from build123d import *

# Parameters (mm, degrees)
F1_DEPTH = 25


with BuildPart() as f1:
    # F0 (on Front) → F1 (new body)
    with BuildSketch(Plane.XZ):
        with BuildLine():
            Line((5, 30.5941170816), (5, 39.686269666))
            ThreePointArc((5, 39.686269666), (2.5049165017, 39.9214903695), (0, 40))
            Line((0, 40), (0, 31))
            ThreePointArc((0, 31), (2.5082235219, 30.8983626551), (5, 30.5941170816))
        make_face()
        with BuildLine():
            Line((0, 31), (0, 40))
            ThreePointArc((0, 40), (-2.5049165017, 39.9214903695), (-5, 39.686269666))
            Line((-5, 39.686269666), (-5, 30.5941170816))
            ThreePointArc((-5, 30.5941170816), (-2.5082235219, 30.8983626551), (0, 31))
        make_face()
        with BuildLine():
            Line((-5, 30.5941170816), (-5, 39.686269666))
            ThreePointArc((-5, 39.686269666), (-28.2842712475, 28.2842712475), (-39.686269666, 5))
            Line((-39.686269666, 5), (-30.5941170816, 5))
            ThreePointArc((-30.5941170816, 5), (-21.9203102168, 21.9203102168), (-5, 30.5941170816))
        make_face()
        with BuildLine():
            Line((-30.5941170816, 5), (-39.686269666, 5))
            ThreePointArc((-39.686269666, 5), (-39.9214903695, 2.5049165017), (-40, 0))
            Line((-40, 0), (-31, 0))
            ThreePointArc((-31, 0), (-30.8983626551, 2.5082235219), (-30.5941170816, 5))
        make_face()
        with BuildLine():
            ThreePointArc((-40, 0), (-39.9214903695, -2.5049165017), (-39.686269666, -5))
            Line((-39.686269666, -5), (-30.5941170816, -5))
            ThreePointArc((-30.5941170816, -5), (-30.8983626551, -2.5082235219), (-31, 0))
            Line((-31, 0), (-40, 0))
        make_face()
        with BuildLine():
            ThreePointArc((-39.686269666, -5), (-28.2842712475, -28.2842712475), (-5, -39.686269666))
            Line((-5, -39.686269666), (-5, -30.5941170816))
            ThreePointArc((-5, -30.5941170816), (-21.9203102168, -21.9203102168), (-30.5941170816, -5))
            Line((-30.5941170816, -5), (-39.686269666, -5))
        make_face()
        with BuildLine():
            ThreePointArc((-5, -39.686269666), (-2.5049165017, -39.9214903695), (0, -40))
            Line((0, -40), (0, -31))
            ThreePointArc((0, -31), (-2.5082235219, -30.8983626551), (-5, -30.5941170816))
            Line((-5, -30.5941170816), (-5, -39.686269666))
        make_face()
        with BuildLine():
            ThreePointArc((0, -40), (2.5049165017, -39.9214903695), (5, -39.686269666))
            Line((5, -39.686269666), (5, -30.5941170816))
            ThreePointArc((5, -30.5941170816), (2.5082235219, -30.8983626551), (0, -31))
            Line((0, -31), (0, -40))
        make_face()
        with BuildLine():
            ThreePointArc((5, -39.686269666), (28.2842712475, -28.2842712475), (39.686269666, -5))
            Line((39.686269666, -5), (30.5941170816, -5))
            ThreePointArc((30.5941170816, -5), (21.9203102168, -21.9203102168), (5, -30.5941170816))
            Line((5, -30.5941170816), (5, -39.686269666))
        make_face()
        with BuildLine():
            ThreePointArc((39.686269666, -5), (39.9214903695, -2.5049165017), (40, 0))
            Line((40, 0), (31, 0))
            ThreePointArc((31, 0), (30.8983626551, -2.5082235219), (30.5941170816, -5))
            Line((30.5941170816, -5), (39.686269666, -5))
        make_face()
        with BuildLine():
            Line((31, 0), (40, 0))
            ThreePointArc((40, 0), (39.9214903695, 2.5049165017), (39.686269666, 5))
            Line((39.686269666, 5), (30.5941170816, 5))
            ThreePointArc((30.5941170816, 5), (30.8983626551, 2.5082235219), (31, 0))
        make_face()
        with BuildLine():
            Line((30.5941170816, 5), (39.686269666, 5))
            ThreePointArc((39.686269666, 5), (28.2842712475, 28.2842712475), (5, 39.686269666))
            Line((5, 39.686269666), (5, 30.5941170816))
            ThreePointArc((5, 30.5941170816), (21.9203102168, 21.9203102168), (30.5941170816, 5))
        make_face()
    extrude(amount=F1_DEPTH)


solid = f1.part
Read the model definition and answer for the solid it produces. Units are mm, in the model's axes. Coordinates: 2 decimals unless noted, no trailing zeros. Order: outer loops, then holes, each group sorted by start corner. A loop starts at its lowest first (then second) coordinate and runs counter-clockwise, first axis right, second up. Notation, with made-up numbers: M -28,-30 L 3,-30 A21 ccw 3,-24 Z; hole C 30,0.25 d1. An arc over 180 degrees is marked long. Put each result on its own line as item: value. Start each with the question number.
Item 1: Section D-D, the plane x = 34 is taken. Determine the outline of the cut face in (y, z).
Item 2: Section C-C, the plane z = 7.5 is taken. Determine the outline of the cut face in (x, y).
Item 3: Section B-B, the plane x = -26 is taken. Determine the outline of the cut face in (y, z).
Item 4: Given pin 1 Ø3 at (x, y) = (-26.5, -5) entering from -Z (3 decimals); pin 2 Ø4 at (y, z) = (-8.5, -28.5) entering from -X; pin 3 Ø10 at (x, y) = (-26.5, -11) entering from -Z, each flat-ended and moving along its own axis, determine where each tip first touches the part or whether it passes through.
Item 5: Section A-A, the plane y = -6.5 is taken. Determine the outline of the cut face in (x, z).
Item 6: Consider probe 1 along X at (y, z) = (-2.75, -9); probe 2 along Z at (x, y) = (-25.5, -3.75); probe 3 along Z at (x, y) = (16, -8.25). Determine where each line is inside the solid, lowest interval first. Write a range as [from, to].
Computed:
1. outline: M -25,-21.07 L 0,-21.07 L 0,21.07 L -25,21.07 Z
2. outline: M -39.29,-25 L -30.08,-25 L -30.08,0 L -39.29,0 Z; M 30.08,-25 L 39.29,-25 L 39.29,0 L 30.08,0 Z
3. outline: M -25,-30.4 L 0,-30.4 L 0,-16.88 L -25,-16.88 Z; M -25,16.88 L 0,16.88 L 0,30.4 L -25,30.4 Z
4. pin 1: stops at z = -31.225
4. pin 2: stops at x = -29.96
4. pin 3: stops at z = -33.73
5. outline: C 0,0 d80; hole C 0,0 d62
6. probe 1: x = [-38.97, -29.66], [29.66, 38.97]
6. probe 2: z = [-30.82, -17.63], [17.63, 30.82]
6. probe 3: z = [-36.66, -26.55], [26.55, 36.66]
